For this review, use the dimensioned drawing (mm, ordinates from the lowest corner) and the shaded views. A direction names the side the tool comes from. Give positions to 0.01 mm unless a question says otherwise; leave off trailing zeros. Order: outer loops, then holes, each group sorted by start corner. A loop starts at its lowest first (then second) coordinate and runs counter-clockwise, first axis right, second up. Notation, with made-up numbers: M 6,53 L 62,53 A26 cw 62,84 Z; hole C -2.5,79.5 d5. An arc over 180 degrees is marked long. Answer as CSV lines item,"result". Start each with the question number.
1. Clearance check with flat-ended pins moving along their axes: P1, Ø0.6, axis at x = 0.5, y = 24.5, coming from the -Z side; P2, Ø1.2, axis at y = 46, z = 11.5, coming from the -X side; P3, Ø4, axis at x = 17.4, z = 15, coming from the +Y side; P4, Ø8, axis at x = 7.5, y = 25, coming from the +Z side. State where each tip first meets the part, or that it passes through.
2. We need section B-B, the plane y = 8.9. Give the boundary of the cut face in (x, z), and give its area (3 significant figures).
3. We need section C-C, the plane x = 25. Give the boundary of the cut face in (y, z), and give its area (3 significant figures).
4. Mouldability with a two-part tool opening along Y and no side actions: class the marked faces 1, 2, 3 and 4 as pulls with the +Y half, pulls with the -Y half, needs draft (parallel to the pull), parting line crosses it, or undercut.
5. For line 1 along Z through (x, y) = (17.4, 47.05); line 2 along X through (y, z) = (12, 26.5); line 3 along Y through (x, z) = (25, 12.5), list the stretches that pass through material, from the lowest coordinate up.
6. Machinability: for the marked faces 5 and 6, which of the approach directions +Z, -Z, +X, -X, +Y, -Y give a long, thin tool a straight path to every point of the face, cutting with its end or side? Answer none if there is none.
7. We need section A-A, the plane x = 17.4. State how many separate pieces and enclosed holes the cut face has, and give its area (3 significant figures).
8. We need section D-D, the plane z = 7.5. Give the boundary of the cut face in (x, y), and give its area (3 significant figures).
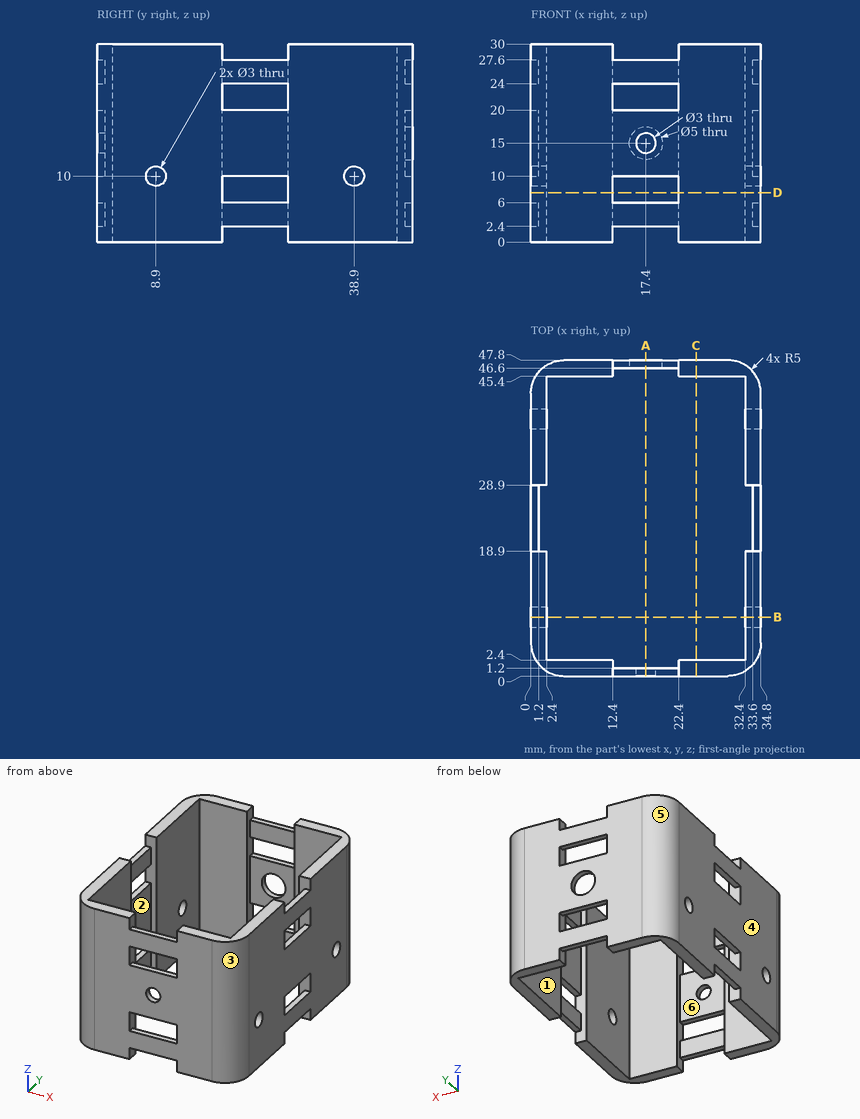
Result set:
1,P1,"z = 2.4"
1,P2,"x = 0.73"
1,P3,"y = 1.2"
1,P4,"through"
2,outline,"M 0,0 L 2.4,0 L 2.4,8.5 L 0,8.5 Z; M 0,11.5 L 2.4,11.5 L 2.4,30 L 0,30 Z; M 32.4,0 L 34.8,0 L 34.8,8.5 L 32.4,8.5 Z; M 32.4,11.5 L 34.8,11.5 L 34.8,30 L 32.4,30 Z"
2,area,"130 mm2"
3,outline,"M 0,0 L 2.4,0 L 2.4,30 L 0,30 Z; M 45.4,0 L 47.8,0 L 47.8,30 L 45.4,30 Z"
3,area,"144 mm2"
4,face 1,"undercut"
4,face 2,"undercut"
4,face 3,"pulls with the -Y half"
4,face 4,"needs draft"
5,line 1,"2.4 to 6, 10 to 12.5, 17.5 to 20, 24 to 27.6"
5,line 2,"0 to 2.4, 32.4 to 34.8"
5,line 3,"0 to 2.4, 45.4 to 47.8"
6,face 5,"+Z, -Z, -X, +Y"
6,face 6,"+Z, -Z"
7,separate pieces,"8"
7,enclosed holes,"0"
7,area,"31.7 mm2"
8,outline,"M 0,5 A5 ccw 5,0 L 12.4,0 L 12.4,2.4 L 2.4,2.4 L 2.4,18.9 L 0,18.9 Z; M 0,28.9 L 2.4,28.9 L 2.4,45.4 L 12.4,45.4 L 12.4,47.8 L 5,47.8 A5 ccw 0,42.8 Z; M 22.4,0 L 29.8,0 A5 ccw 34.8,5 L 34.8,18.9 L 32.4,18.9 L 32.4,2.4 L 22.4,2.4 Z; M 22.4,45.4 L 32.4,45.4 L 32.4,28.9 L 34.8,28.9 L 34.8,42.8 A5 ccw 29.8,47.8 L 22.4,47.8 Z"
8,area,"256 mm2"
